from build123d import *

# Parameters (mm, degrees)
SKETCH_1_W          = 125
SKETCH_1_H          = 23.5
EXTRUDE_1_DEPTH     = 1.5
CUT_EXTRUDE_1_DEPTH = 64.612597023


with BuildPart() as part:
    # Эскиз1 → Бобышка-Вытянуть1 (new body)
    with BuildSketch(Plane(origin=(0, 0, 0), x_dir=(1, 0, 0), z_dir=(0, 1, 0))):
        Rectangle(SKETCH_1_W, SKETCH_1_H)
    extrude(amount=EXTRUDE_1_DEPTH)

    # Эскиз2 → Вырез-Вытянуть1 (cut, through all)
    with BuildSketch(Plane(origin=(0, 1.5, 0), x_dir=(1, 0, 0), z_dir=(0, 1, 0))):
        with BuildLine():
            ThreePointArc((62.5, 11), (60.629171307, 9.707106781), (61.177124344, 7.5))
            ThreePointArc((61.177124344, 7.5), (61.792893219, 7.870828693), (62.5, 8))
            Line((62.5, 8), (62.5, 11))
        make_face()
        with BuildLine():
            ThreePointArc((62.5, 8), (61.792893219, 7.870828693), (61.177124344, 7.5))
            ThreePointArc((61.177124344, 7.5), (61.792893219, 7.129171307), (62.5, 7))
            Line((62.5, 7), (62.5, 8))
        make_face()
        with BuildLine():
            Line((62.5, 8), (62.5, 7))
            ThreePointArc((62.5, 7), (63.207106781, 7.129171307), (63.822875656, 7.5))
            ThreePointArc((63.822875656, 7.5), (63.207106781, 7.870828693), (62.5, 8))
        make_face()
        with BuildLine():
            ThreePointArc((62.5, 8), (63.207106781, 7.870828693), (63.822875656, 7.5))
            ThreePointArc((63.822875656, 7.5), (64.322875656, 8.177124344), (64.5, 9))
            ThreePointArc((64.5, 9), (63.914213562, 10.414213562), (62.5, 11))
            Line((62.5, 11), (62.5, 8))
        make_face()
        with BuildLine():
            ThreePointArc((62.5, 5), (63.207106781, 4.870828693), (63.822875656, 4.5))
            ThreePointArc((63.822875656, 4.5), (64.322875656, 5.177124344), (64.5, 6))
            ThreePointArc((64.5, 6), (64.322875656, 6.822875656), (63.822875656, 7.5))
            ThreePointArc((63.822875656, 7.5), (63.207106781, 7.129171307), (62.5, 7))
            Line((62.5, 7), (62.5, 5))
        make_face()
        with BuildLine():
            ThreePointArc((61.177124344, 7.5), (60.5, 6), (61.177124344, 4.5))
            ThreePointArc((61.177124344, 4.5), (61.792893219, 4.870828693), (62.5, 5))
            Line((62.5, 5), (62.5, 7))
            ThreePointArc((62.5, 7), (61.792893219, 7.129171307), (61.177124344, 7.5))
        make_face()
        with BuildLine():
            Line((62.5, 5), (62.5, 4))
            ThreePointArc((62.5, 4), (63.207106781, 4.129171307), (63.822875656, 4.5))
            ThreePointArc((63.822875656, 4.5), (63.207106781, 4.870828693), (62.5, 5))
        make_face()
        with BuildLine():
            ThreePointArc((61.177124344, 4.5), (61.792893219, 4.129171307), (62.5, 4))
            Line((62.5, 4), (62.5, 5))
            ThreePointArc((62.5, 5), (61.792893219, 4.870828693), (61.177124344, 4.5))
        make_face()
        with BuildLine():
            ThreePointArc((62.5, 2), (63.207106781, 1.870828693), (63.822875656, 1.5))
            ThreePointArc((63.822875656, 1.5), (64.322875656, 2.177124344), (64.5, 3))
            ThreePointArc((64.5, 3), (64.322875656, 3.822875656), (63.822875656, 4.5))
            ThreePointArc((63.822875656, 4.5), (63.207106781, 4.129171307), (62.5, 4))
            Line((62.5, 4), (62.5, 2))
        make_face()
        with BuildLine():
            ThreePointArc((61.177124344, 1.5), (61.792893219, 1.870828693), (62.5, 2))
            Line((62.5, 2), (62.5, 4))
            ThreePointArc((62.5, 4), (61.792893219, 4.129171307), (61.177124344, 4.5))
            ThreePointArc((61.177124344, 4.5), (60.5, 3), (61.177124344, 1.5))
        make_face()
        with BuildLine():
            ThreePointArc((62.5, 1), (63.207106781, 1.129171307), (63.822875656, 1.5))
            ThreePointArc((63.822875656, 1.5), (63.207106781, 1.870828693), (62.5, 2))
            Line((62.5, 2), (62.5, 1))
        make_face()
        with BuildLine():
            Line((62.5, 1), (62.5, 2))
            ThreePointArc((62.5, 2), (61.792893219, 1.870828693), (61.177124344, 1.5))
            ThreePointArc((61.177124344, 1.5), (61.792893219, 1.129171307), (62.5, 1))
        make_face()
        with BuildLine():
            ThreePointArc((63.822875656, -1.5), (64.322875656, -0.822875656), (64.5, 0))
            ThreePointArc((64.5, 0), (64.322875656, 0.822875656), (63.822875656, 1.5))
            ThreePointArc((63.822875656, 1.5), (63.207106781, 1.129171307), (62.5, 1))
            Line((62.5, 1), (62.5, -1))
            ThreePointArc((62.5, -1), (63.207106781, -1.129171307), (63.822875656, -1.5))
        make_face()
        with BuildLine():
            Line((62.5, -1), (62.5, 1))
            ThreePointArc((62.5, 1), (61.792893219, 1.129171307), (61.177124344, 1.5))
            ThreePointArc((61.177124344, 1.5), (60.5, 0), (61.177124344, -1.5))
            ThreePointArc((61.177124344, -1.5), (61.792893219, -1.129171307), (62.5, -1))
        make_face()
        with BuildLine():
            ThreePointArc((62.5, -2), (63.207106781, -1.870828693), (63.822875656, -1.5))
            ThreePointArc((63.822875656, -1.5), (63.207106781, -1.129171307), (62.5, -1))
            Line((62.5, -1), (62.5, -2))
        make_face()
        with BuildLine():
            ThreePointArc((61.177124344, -1.5), (61.792893219, -1.870828693), (62.5, -2))
            Line((62.5, -2), (62.5, -1))
            ThreePointArc((62.5, -1), (61.792893219, -1.129171307), (61.177124344, -1.5))
        make_face()
        with BuildLine():
            ThreePointArc((64.5, -3), (64.322875656, -2.177124344), (63.822875656, -1.5))
            ThreePointArc((63.822875656, -1.5), (63.207106781, -1.870828693), (62.5, -2))
            Line((62.5, -2), (62.5, -4))
            ThreePointArc((62.5, -4), (63.207106781, -4.129171307), (63.822875656, -4.5))
            ThreePointArc((63.822875656, -4.5), (64.322875656, -3.822875656), (64.5, -3))
        make_face()
        with BuildLine():
            Line((62.5, -4), (62.5, -2))
            ThreePointArc((62.5, -2), (61.792893219, -1.870828693), (61.177124344, -1.5))
            ThreePointArc((61.177124344, -1.5), (60.5, -3), (61.177124344, -4.5))
            ThreePointArc((61.177124344, -4.5), (61.792893219, -4.129171307), (62.5, -4))
        make_face()
        with BuildLine():
            Line((62.5, -5), (62.5, -4))
            ThreePointArc((62.5, -4), (61.792893219, -4.129171307), (61.177124344, -4.5))
            ThreePointArc((61.177124344, -4.5), (61.792893219, -4.870828693), (62.5, -5))
        make_face()
        with BuildLine():
            ThreePointArc((63.822875656, -4.5), (63.207106781, -4.129171307), (62.5, -4))
            Line((62.5, -4), (62.5, -5))
            ThreePointArc((62.5, -5), (63.207106781, -4.870828693), (63.822875656, -4.5))
        make_face()
        with BuildLine():
            ThreePointArc((64.5, -6), (64.322875656, -5.177124344), (63.822875656, -4.5))
            ThreePointArc((63.822875656, -4.5), (63.207106781, -4.870828693), (62.5, -5))
            Line((62.5, -5), (62.5, -7))
            ThreePointArc((62.5, -7), (63.207106781, -7.129171307), (63.822875656, -7.5))
            ThreePointArc((63.822875656, -7.5), (64.322875656, -6.822875656), (64.5, -6))
        make_face()
        with BuildLine():
            ThreePointArc((62.5, -5), (61.792893219, -4.870828693), (61.177124344, -4.5))
            ThreePointArc((61.177124344, -4.5), (60.5, -6), (61.177124344, -7.5))
            ThreePointArc((61.177124344, -7.5), (61.792893219, -7.129171307), (62.5, -7))
            Line((62.5, -7), (62.5, -5))
        make_face()
        with BuildLine():
            ThreePointArc((62.5, -7), (61.792893219, -7.129171307), (61.177124344, -7.5))
            ThreePointArc((61.177124344, -7.5), (61.792893219, -7.870828693), (62.5, -8))
            Line((62.5, -8), (62.5, -7))
        make_face()
        with BuildLine():
            ThreePointArc((62.5, -8), (61.792893219, -7.870828693), (61.177124344, -7.5))
            ThreePointArc((61.177124344, -7.5), (60.629171307, -9.707106781), (62.5, -11))
            Line((62.5, -11), (62.5, -8))
        make_face()
        with BuildLine():
            ThreePointArc((63.822875656, -7.5), (63.207106781, -7.129171307), (62.5, -7))
            Line((62.5, -7), (62.5, -8))
            ThreePointArc((62.5, -8), (63.207106781, -7.870828693), (63.822875656, -7.5))
        make_face()
        with BuildLine():
            ThreePointArc((64.5, -9), (64.322875656, -8.177124344), (63.822875656, -7.5))
            ThreePointArc((63.822875656, -7.5), (63.207106781, -7.870828693), (62.5, -8))
            Line((62.5, -8), (62.5, -11))
            ThreePointArc((62.5, -11), (63.914213562, -10.414213562), (64.5, -9))
        make_face()
    extrude(amount=-CUT_EXTRUDE_1_DEPTH, mode=Mode.SUBTRACT)


solid = part.part
Could you check a few things on this model? Use its own coordinates, in mm. Give positions to 0.01 mm unless a question says otherwise; leave off trailing zeros. Order: outer loops, then holes, each group sorted by start corner. A loop starts at its lowest first (then second) coordinate and runs counter-clockwise, first axis right, second up.
1. Suppose I cut it at B-B (z = 5.75). List the corners of the cut face in (x, y) for me, plus the area to 3 significant figures.
2. We'd pull the mould along Z, two halves only. Please class faces 1 (the cylindrical face through (60.64, 0.76, -9.74)), 2 (the flat face through (-1, 1.5, 0)): pulls with the +Z half, pulls with the -Z half, needs draft (parallel to the pull), parting line crosses it, or undercut.
3. Suppose I cut it at A-A (z = -9.5). List the corners of the cut face in (x, y) for me.
4. I need wall thicknesses on L1, parallel to X at y = 1, z = 8.75; L2, parallel to X at y = 0.2, z = -6.5. Which ranges of each line are inside material? Lowest first, please.
Solved:
1. outline: (-62.5, 0) - (60.52, 0) - (60.52, 1.5) - (-62.5, 1.5) - close
1. area: 185 mm2
2. face 1: undercut
2. face 2: needs draft
3. outline: (-62.5, 0) - (60.56, 0) - (60.56, 1.5) - (-62.5, 1.5) - close
4. L1: x = -62.5 to 60.52
4. L2: x = -62.5 to 60.56
